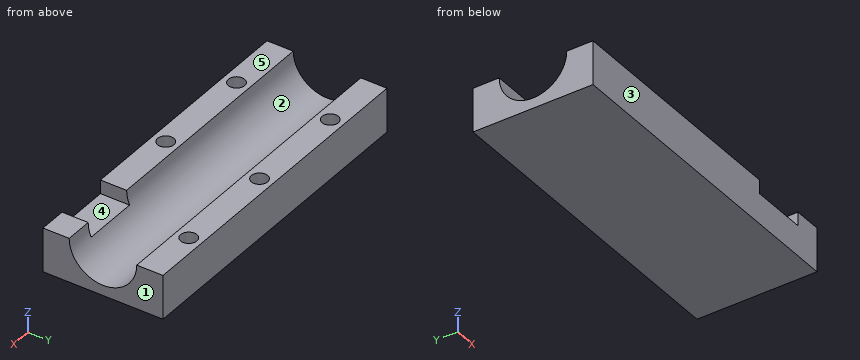
```python
from build123d import *

# Parameters (mm, degrees)
SKETCH1_W                = 118.11
SKETCH1_H                = 44.45
BOSS_EXTRUDE1_DEPTH      = 2
BOSS_EXTRUDE2_DEPTH      = 2.54
BOSS_EXTRUDE2_DEPTH_BACK = 118.11
SKETCH3_R                = 3.025
CUT_EXTRUDE1_DEPTH       = 8
SKETCH11_W               = 20.708368279
SKETCH11_H               = 9.6981
CUT_EXTRUDE4_DEPTH       = 5.08
SKETCH12_W               = 20.708368279
SKETCH12_H               = 5.08
CUT_EXTRUDE5_DEPTH       = 2.54
LPATTERN1_COUNT          = 2
LPATTERN1_PITCH          = 38.1
MIRROR1_COPY_1_SKETCH_R  = 3.025
MIRROR1_COPY_1_DEPTH     = 8
LPATTERN2_COUNT          = 2
LPATTERN2_PITCH          = 38.1
SKETCH16_W               = 2
SKETCH16_H               = 44.45
BOSS_EXTRUDE5_DEPTH      = 2.54


with BuildPart() as part:
    # Sketch1 → Boss-Extrude1 (new body)
    with BuildSketch(Plane.XY):
        Rectangle(SKETCH1_W, SKETCH1_H)
    extrude(amount=BOSS_EXTRUDE1_DEPTH)

    # Sketch2 → Boss-Extrude2 (add, two sides: drawn at the far end of the back side and taken through both)
    with BuildSketch(Plane.ZY.offset(59.055).offset(-BOSS_EXTRUDE2_DEPTH_BACK)):
        with BuildLine():
            Line((16.3195, 22.225), (2, 22.225))
            Line((2, 22.225), (2, -22.225))
            Line((2, -22.225), (16.3195, -22.225))
            Line((16.3195, -22.225), (16.3195, -12.5269))
            ThreePointArc((16.3195, -12.5269), (3.7926, 0), (16.3195, 12.5269))
            Line((16.3195, 12.5269), (16.3195, 22.225))
        make_face()
    extrude(amount=BOSS_EXTRUDE2_DEPTH + BOSS_EXTRUDE2_DEPTH_BACK)

    # Sketch3 → Cut-Extrude1 (cut)
    with BuildSketch(Plane.XY.offset(16.3195)):
        with Locations((0, 17.37595)):
            Circle(SKETCH3_R)
    cut_extrude1 = extrude(amount=-CUT_EXTRUDE1_DEPTH, mode=Mode.SUBTRACT)

    # Sketch11 → Cut-Extrude4 (cut)
    with BuildSketch(Plane.XY.offset(16.3195)):
        with Locations((38.470435787, -17.37595)):
            Rectangle(SKETCH11_W, SKETCH11_H)
    extrude(amount=-CUT_EXTRUDE4_DEPTH, mode=Mode.SUBTRACT)

    # Sketch12 → Cut-Extrude5 (cut)
    with BuildSketch(Plane.XZ.offset(12.5269)):
        with Locations((38.470435787, 13.7795)):
            Rectangle(SKETCH12_W, SKETCH12_H)
    extrude(amount=-CUT_EXTRUDE5_DEPTH, mode=Mode.SUBTRACT)

    # LPattern1: Cut-Extrude1 ×2
    with Locations(*[(-i * LPATTERN1_PITCH, 0, 0) for i in range(1, LPATTERN1_COUNT)]):
        add(cut_extrude1, mode=Mode.SUBTRACT)

    # Mirror1: Cut-Extrude1 across plane
    add(cut_extrude1.mirror(Plane.ZX), mode=Mode.SUBTRACT)

    # Mirror1 copy 1 sketch → Mirror1 copy 1 (cut)
    with BuildSketch(Plane(origin=(-38.1, 0, 16.3195), x_dir=(1, 0, 0), z_dir=(0, 0, 1))):
        with Locations((0, -17.37595)):
            Circle(MIRROR1_COPY_1_SKETCH_R)
    extrude(amount=-MIRROR1_COPY_1_DEPTH, mode=Mode.SUBTRACT)

    # LPattern2: Cut-Extrude1 ×2
    with Locations(*[(i * LPATTERN2_PITCH, 0, 0) for i in range(1, LPATTERN2_COUNT)]):
        add(cut_extrude1, mode=Mode.SUBTRACT)

    # Sketch16 → Boss-Extrude5 (add)
    with BuildSketch(Plane.ZY.offset(59.055)):
        with Locations((1, 0)):
            Rectangle(SKETCH16_W, SKETCH16_H)
    extrude(amount=BOSS_EXTRUDE5_DEPTH)


solid = part.part
```
Geometry: final body of the model. Coordinates: model frame, mm. Face numbers are marked on the shaded views. A direction names the side the tool comes from. Give positions to 0.01 mm unless a question says otherwise; leave off trailing zeros. Order: outer loops, then holes, each group sorted by start corner. A loop starts at its lowest first (then second) coordinate and runs counter-clockwise, first axis right, second up. Notation, with made-up numbers: M -37.75,12 L -30.75,12 A14 cw -30.75,24 Z; hole C 31,85.25 d6. An arc over 180 degrees is marked long. Answer as CSV lines item,"result". Start each with the question number.
1) Cut plane D-D (x = 38.1). Output: boundary loops of the cut face in (y, z) (1 decimal).
2) First-contact query: P1, Ø3, axis at x = -0.5, y = -18.5, coming from the +Z side; P2, Ø3, axis at x = 36, y = -5, coming from the -Z side; P3, Ø5.5, axis at x = 36, y = -19.5, coming from the +Z side. Flat tips, straight axial feed; report the tip coordinate or a pass-through.
3) Set-up query: the marked faces 4 and 5. Return all of +Z, -Z, +X, -X, +Y, -Y with unobstructed straight access to the full face (end or side cutting, diameter ignored); none if empty.
4) Cut plane C-C (y = 0). Output: boundary loops of the cut face in (x, z) (3 decimals).
5) Line query: line 1 (X direction, y = 17, z = 14.5) (3 decimals); line 2 (Y direction, x = -38.1, z = 10.5) (3 decimals); line 3 (X direction, y = -20, z = 15.5) (3 decimals). Output: solid intervals per line, ascending. Write a range as from..to.
6) Mould query, pull axis Y, two halves, no side actions, for the marked faces 1, 2 and 3. Classes: +Y half, -Y half, draft (parallel to the pull), parting line (faces both ways), or undercut.
7) Cut plane B-B (x = -38.1). Output: boundary loops of the cut face in (y, z) (1 decimal), then the cut area to 3 significant figures.
8) Cut plane A-A (z = 15). Output: boundary loops of the cut face in (x, y) (3 decimals), then the cut area to 3 significant figures.
Findings below:
1,outline,"M -22.2,0 L 22.2,0 L 22.2,16.3 L 20.4,16.3 L 20.4,8.3 L 14.4,8.3 L 14.4,16.3 L 12.5,16.3 A12.5 cw -11.5,11.2 L -22.2,11.2 Z"
2,P1,"stops at z = 8.32"
2,P2,"stops at z = 0"
2,P3,"stops at z = 11.24"
3,face 4,"+Z, -Y"
3,face 5,"+Z, +X, -X, +Y, -Y"
4,outline,"M -61.595,0 L 59.055,0 L 59.055,3.793 L -61.595,3.793 Z"
5,line 1,"x = -61.595..-41.102, -35.098..-3.002, 3.002..35.098, 41.102..59.055"
5,line 2,"y = -22.225..-20.401, -14.351..-11.093, 11.093..14.351, 20.401..22.225"
5,line 3,"x = -61.595..-39.605, -36.595..-1.505, 1.505..28.116, 48.825..59.055"
6,face 1,"draft"
6,face 2,"undercut"
6,face 3,"-Y half"
7,outline,"M -22.2,0 L 22.2,0 L 22.2,16.3 L 20.4,16.3 L 20.4,8.3 L 14.4,8.3 L 14.4,16.3 L 12.5,16.3 A12.5 cw -12.5,16.3 L -14.4,16.3 L -14.4,8.3 L -20.4,8.3 L -20.4,16.3 L -22.2,16.3 Z"
7,area,"382 mm²"
8,outline,"M -61.595,-22.225 L 28.116,-22.225 L 28.116,-12.457 L -61.595,-12.457 Z; M -61.595,12.457 L 59.055,12.457 L 59.055,22.225 L -61.595,22.225 Z; M 48.825,-22.225 L 59.055,-22.225 L 59.055,-12.457 L 48.825,-12.457 Z; hole C -38.1,-17.376 d6.05; hole C -38.1,17.376 d6.05; hole C 0,-17.376 d6.05; hole C 0,17.376 d6.05; hole C 38.1,17.376 d6.05"
8,area,"2,010 mm²"
